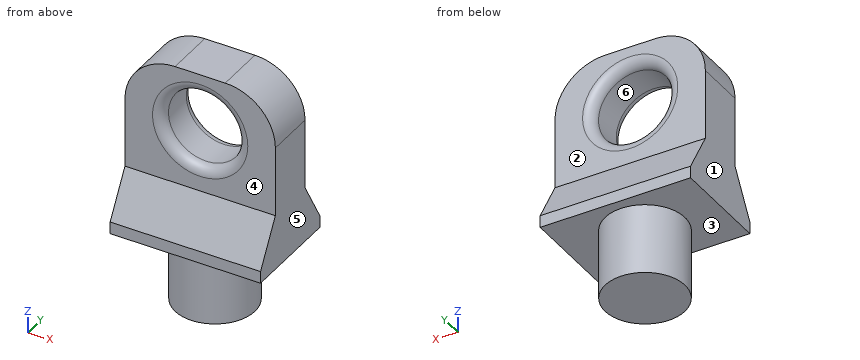
from build123d import *

# Parameters (mm, degrees)
F0_W          = 5.0546
F0_H          = 8.89
F3_DEPTH      = 9.525
F4_R          = 6.35
F5_R          = 4.7625
F6_DEPTH      = 6.351
F6_DEPTH_BACK = 6.351
F7_R          = 1.27


with BuildPart() as f1:
    # F0 (on Front) → F1 (revolve)
    with BuildSketch(Plane.XZ):
        with Locations((2.5273, -4.445)):
            Rectangle(F0_W, F0_H)
    revolve(axis=Axis((0, 0, -4.445), (0, 0, 1)))

    # F2 (on Right) → F3 (join, symmetric)
    with BuildSketch(Plane.YZ):
        Polygon((-6.35, 1.524), (-6.35, 0), (6.35, 0), (6.35, 1.524), (3.175, 7.023261), (3.175, 22.263261), (-3.175, 22.263261), (-3.175, 7.023261), align=None)
    extrude(amount=F3_DEPTH, both=True)

    # F4
    f4_edges = [f1.edges().sort_by_distance(p)[0] for p in [
        (9.525, 0, 22.263261),
        (-9.525, 0, 22.263261),
    ]]
    fillet(f4_edges, radius=F4_R)

    # F5 (on Front) → F6 (cut, two sides)
    with BuildSketch(Plane.XZ) as f6_sk:
        with Locations((0, 14.960761)):
            Circle(F5_R)
    extrude(amount=F6_DEPTH, mode=Mode.SUBTRACT)
    extrude(f6_sk.sketch, amount=-F6_DEPTH_BACK, mode=Mode.SUBTRACT)

    # F7
    f7_edges = [f1.edges().sort_by_distance(p)[0] for p in [
        (-4.7625, -3.175, 14.960761),
        (-4.7625, 3.175, 14.960761),
    ]]
    fillet(f7_edges, radius=F7_R)


solid = f1.part
Part model, mm, in its own coordinate system. Face numbers are marked on the shaded views. A direction names the side the tool comes from. Give positions to 0.01 mm unless a question says otherwise; leave off trailing zeros. Order: outer loops, then holes, each group sorted by start corner. A loop starts at its lowest first (then second) coordinate and runs counter-clockwise, first axis right, second up. Notation, with made-up numbers: (33.25, 54) - (70.25, 54) arc R29 cw to (70.25, 76) - close; hole circle Ø9 at (35.25, 8). An arc over 180 degrees is marked (long way). Use a Markdown table: item, result.
1) Two-plate mould, pull along X, no slides. Class the marked faces 4, 5 and 6: +X half, -X half, draft (parallel to the pull), parting line (faces both ways), or undercut.
Checked values:
| item | result |
|---|---|
| face 4 | draft |
| face 5 | +X half |
| face 6 | undercut |
2) Saw through at D-D on y = 5.75. List the corners of the cut face in (x, z) (3 decimals), plus the area to 3 significant figures.
Checked values:
| item | result |
|---|---|
| outline | (-9.525, 0) - (9.525, 0) - (9.525, 2.563) - (-9.525, 2.563) - close |
| area | 48.8 mm² |
3) Saw through at C-C on x = -7. List the corners of the cut face in (y, z) (3 decimals).
Checked values:
| item | result |
|---|---|
| outline | (-6.35, 0) - (6.35, 0) - (6.35, 1.524) - (3.175, 7.023) - (3.175, 20.982) - (-3.175, 20.982) - (-3.175, 7.023) - (-6.35, 1.524) - close |
4) Probe L1, parallel to Z at x = 0, y = 0.6; L2, parallel to Y at x = 7.75, z = 19 (3 decimals); L3, parallel to Z at x = 0.75, y = 2.5. List the from-to ranges inside material, lowest first. Write a range as from..to.
Checked values:
| item | result |
|---|---|
| L1 | -8.89..10.2, 19.72..22.26 |
| L2 | -3.175..3.175 |
| L3 | -8.89..10.11, 19.81..22.26 |
5) 3-axis set-ups, long thin cutter, end or side, ignore diameter. For the marked faces 1, 2 and 3: which of +Z, -Z, +X, -X, +Y, -Y reach the whole face in a straight line?
Checked values:
| item | result |
|---|---|
| face 1 | +Z, -Z, -X, +Y, -Y |
| face 2 | +Z, +X, -X, +Y |
| face 3 | -Z |
6) Saw through at A-A on x = 0. List the corners of the cut face in (y, z) (3 decimals), plus the area to 3 significant figures.
Checked values:
| item | result |
|---|---|
| outline | (-6.35, 0) - (-5.055, 0) - (-5.055, -8.89) - (5.055, -8.89) - (5.055, 0) - (6.35, 0) - (6.35, 1.524) - (3.175, 7.023) - (3.175, 8.928) arc R1.27 ccw to (1.905, 10.198) - (-1.905, 10.198) arc R1.27 ccw to (-3.175, 8.928) - (-3.175, 7.023) - (-6.35, 1.524) - close; (-3.175, 20.993) arc R1.27 ccw to (-1.905, 19.723) - (1.905, 19.723) arc R1.27 ccw to (3.175, 20.993) - (3.175, 22.263) - (-3.175, 22.263) - close |
| area | 197 mm² |
7) Flat gauge pins, fed straight in: P1, Ø4.5, axis at x = 0, z = 17, coming from the -Y side; P2, Ø1.5, axis at x = 7, z = 14, coming from the +Y side (3 decimals); P3, Ø1.5, axis at x = 6, z = 2.5, coming from the +Y side. Where does each tip first touch, or does it go through?
Checked values:
| item | result |
|---|---|
| P1 | through |
| P2 | y = 3.175 |
| P3 | y = 6.22 |
